Here's the drawing with two shaded views (mm, measured from the low corner). I have some questions. A direction names the side the tool comes from. Round coordinates to 2 decimals unless told otherwise and drop trailing zeros. Order: outer loops, then holes, each group sorted by start corner. A loop starts at its lowest first (then second) coordinate and runs counter-clockwise, first axis right, second up.
Q1. If we section it at A-A (z = 13.5): Please give me the cut outline in (x, y), plus the area to 3 significant figures.
Q2. For the marked faces 4, 5 and 6, which set-ups out of +Z, -Z, +X, -X, +Y, -Y let a thin tool reach every point of the face, with its end or its side?
Q3. If we section it at D-D (z = 19.5): Please give me the cut outline in (x, y).
Q4. Will these pins go through, and if not, where does the flat tip stop? P1, Ø3, axis at x = 41, z = 4.5, coming from the -Y side; P2, Ø7.5, axis at y = 9, z = 6, coming from the +X side; P3, Ø8, axis at x = 58.5, y = 50, coming from the +Z side.
Q5. If we section it at C-C (y = 21): Please give me the cut outline in (x, z), plus the area to 3 significant figures.
Q6. If we section it at B-B (x = 42): Please give me the cut outline in (y, z) (3 decimals), plus the area to 3 significant figures.
Q7. We'd pull the mould along X, two halves only. Please class the marked faces 1, 2 and 3: pulls with the +X half, pulls with the -X half, needs draft (parallel to the pull), parting line crosses it, or undercut.
Q8. If I drill on line 1 (Y direction, x = 17.5, z = 38); line 2 (Y direction, x = 37, z = 8); line 3 (Z direction, x = 22, y = 52), over which ranges is the centre line in solid material (lowest first)?
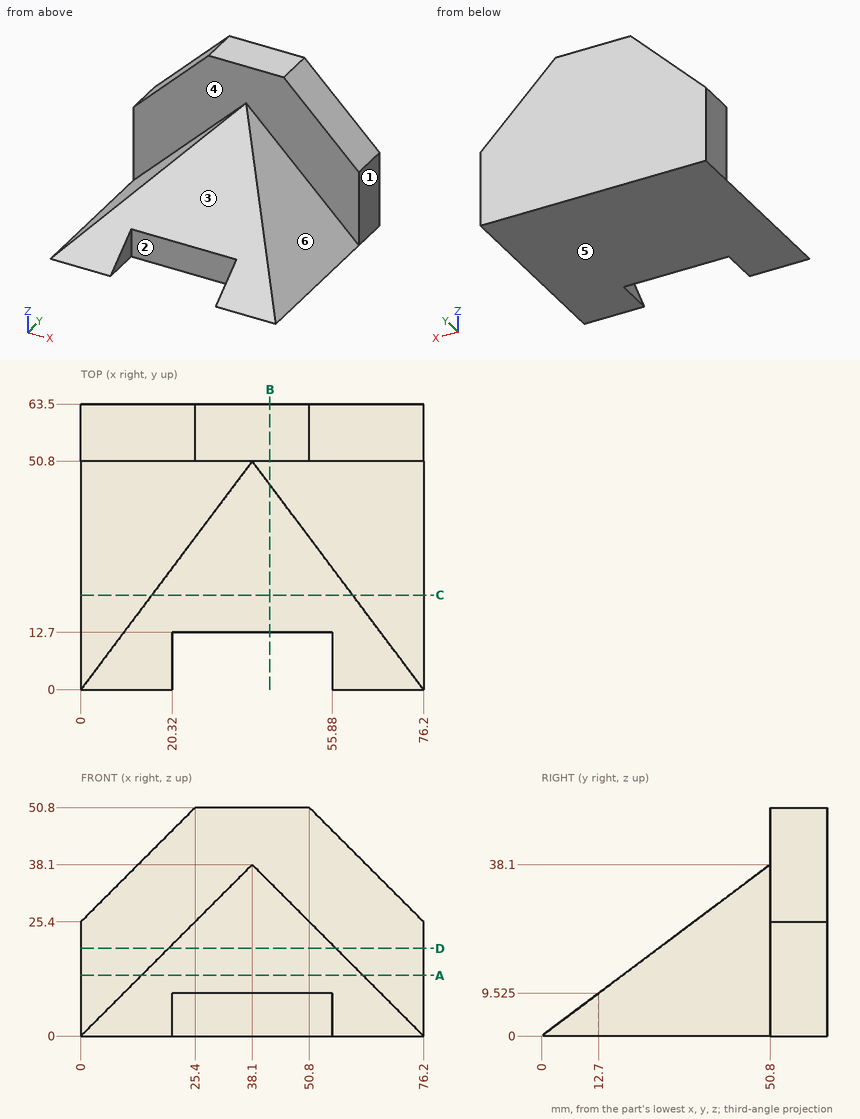
Solution:
1. outline: (0, 50.8) - (13.5, 50.8) - (13.5, 18) - (62.7, 18) - (62.7, 50.8) - (76.2, 50.8) - (76.2, 63.5) - (0, 63.5) - close
1. area: 2,580 mm2
2. face 4: +Z, -Y
2. face 5: -Z, +X, -X, +Y, -Y
2. face 6: +Z, +X, -Y
3. outline: (0, 50.8) - (19.5, 50.8) - (19.5, 26) - (56.7, 26) - (56.7, 50.8) - (76.2, 50.8) - (76.2, 63.5) - (0, 63.5) - close
4. P1: stops at y = 12.7
4. P2: stops at x = 73.95
4. P3: stops at z = 47.02
5. outline: (0, 0) - (76.2, 0) - (60.45, 15.75) - (15.75, 15.75) - close
5. area: 952 mm2
6. outline: (12.7, 0) - (63.5, 0) - (63.5, 50.8) - (50.8, 50.8) - (50.8, 34.2) - (45.6, 34.2) - (12.7, 9.525) - close
6. area: 1,540 mm2
7. face 1: pulls with the +X half
7. face 2: undercut
7. face 3: needs draft
8. line 1: y = 50.8 to 63.5
8. line 2: y = 12.7 to 63.5
8. line 3: z = 0 to 47.4
